```python
from build123d import *

# Parameters (mm, degrees)
SKETCH1_R           = 3.175
BOSS_EXTRUDE1_DEPTH = 3.175


with BuildPart() as part:
    # Sketch1 → Boss-Extrude1 (new body)
    with BuildSketch(Plane.XY):
        with BuildLine():
            ThreePointArc((0, 7.9502), (-5.621640332, 5.621640332), (-7.9502, 0))
            Line((-7.9502, 0), (-12.525754193, -55.05345954))
            Line((-12.525754193, -55.05345954), (-12.7, -57.15))
            ThreePointArc((-12.7, -57.15), (0, -69.85), (12.7, -57.15))
            Line((12.7, -57.15), (12.525900071, -55.054331273))
            Line((12.525900071, -55.054331273), (9.183881789, -14.825922015))
            ThreePointArc((9.183881789, -14.825922015), (10.839778656, -9.999957844), (15.512081878, -7.9502))
            Line((15.512081878, -7.9502), (34.925, -7.9502))
            ThreePointArc((34.925, -7.9502), (42.8752, 0), (34.925, 7.9502))
            Line((34.925, 7.9502), (0, 7.9502))
        make_face()
        with Locations((0, -57.15)):
            Circle(SKETCH1_R, mode=Mode.SUBTRACT)
        Circle(SKETCH1_R, mode=Mode.SUBTRACT)
        with Locations((34.925, 0)):
            Circle(SKETCH1_R, mode=Mode.SUBTRACT)
    extrude(amount=BOSS_EXTRUDE1_DEPTH)


solid = part.part
```
Could you check a few things on this model? Use its own coordinates, in mm. Round coordinates to 2 decimals unless told otherwise and drop trailing zeros. Loops run counter-clockwise (first coordinate to the right, second up) from the corner with the lowest first, then second, coordinate; pieces in that order, holes last. Notation, with made-up numbers: M -11.5,-16 L 31.5,-16 A13 ccw 31.5,5 Z; hole C 75.25,-4.75 d4. An arc over 180 degrees is marked long. Answer as CSV lines item,"result".
1) Imagine slicing it at B-B on x = 10. List the corners of the cut face in (y, z) for me (3 decimals), and give its area (3 significant figures).
From the geometry:
outline,"M -64.979,0 L -24.65,0 L -24.65,3.175 L -64.979,3.175 Z; M -11.148,0 L 7.95,0 L 7.95,3.175 L -11.148,3.175 Z"
area,"189 mm^2"
2) Imagine slicing it at C-C on x = 19. List the corners of the cut face in (y, z) for me (3 decimals), and give its area (3 significant figures).
From the geometry:
outline,"M -7.95,0 L 7.95,0 L 7.95,3.175 L -7.95,3.175 Z"
area,"50.5 mm^2"
3) For pin 1 Ø7.5 at (x, y) = (0, -57.15) entering from +Z (3 decimals); pin 2 Ø5 at (x, y) = (0, 0) entering from +Z; pin 3 Ø1.6 at (x, z) = (21.5, 1) entering from -Y, each with a flat end and sliding along its axis, tell me the tip position at first contact or that it passes through.
From the geometry:
pin 1,"z = 3.175"
pin 2,"through"
pin 3,"y = -7.95"
4) If I drill on probe 1 along Y at (x, z) = (0, 1.5) (3 decimals); probe 2 along X at (y, z) = (-2, 0.95); probe 3 along Y at (x, z) = (29, 0.35), over which ranges is the centre line in solid material (lowest first)?
From the geometry:
probe 1,"-69.85 to -60.325, -53.975 to -3.175, 3.175 to 7.95"
probe 2,"-8.12 to -2.47, 2.47 to 32.46, 37.39 to 42.62"
probe 3,"-7.95 to 7.95"
5) We'd pull the mould along Y, two halves only. Please class faces 1 (the cylindrical face through (-0.69, -3.1, 1.57)), 2 (the cylindrical face through (-5.56, 5.68, 1.57)), 3 (the flat face through (25, -7.95, 2)): released by +Y, released by -Y, zero draft, split by the parting line, or undercut.
From the geometry:
face 1,"undercut"
face 2,"released by +Y"
face 3,"released by -Y"
6) Imagine slicing it at D-D on y = -34. List the corners of the cut face in (x, z) for me (3 decimals).
From the geometry:
outline,"M -10.776,0 L 10.777,0 L 10.777,3.175 L -10.776,3.175 Z"
7) Imagine slicing it at A-A on y = -59. List the corners of the cut face in (x, z) for me (3 decimals), and give its area (3 significant figures).
From the geometry:
outline,"M -12.565,0 L -2.58,0 L -2.58,3.175 L -12.565,3.175 Z; M 2.58,0 L 12.565,0 L 12.565,3.175 L 2.58,3.175 Z"
area,"63.4 mm^2"
